from build123d import *

# Parameters (mm, degrees)
SKETCH1_R           = 2.1
BOSS_EXTRUDE1_DEPTH = 1500
FILLET1_R           = 0.5


with BuildPart() as part:
    # Sketch1 → Boss-Extrude1 (new body)
    with BuildSketch(Plane.XY):
        Polygon((-20, -10), (-15.5, -10), (-15.1, -10), (-13.1, -8), (-15.5, -8), (-15.5, -6.560660172), (-12.539339828, -3.6), (-7.460660172, -3.6), (-4.5, -6.560660172), (-4.5, -8), (-6.9, -8), (-4.9, -10), (5.313777138, -10), (7.313777138, -8), (4.5, -8), (4.5, -6.560660172), (7.460660172, -3.6), (12.539339828, -3.6), (15.5, -6.560660172), (15.5, -8), (13.513777138, -8), (15.1, -10), (15.5, -10), (20, -10), (20, -5.5), (20, -5.1), (18, -3.1), (18, -5.5), (16.560660172, -5.5), (13.6, -2.539339828), (13.6, 2.539339828), (16.560660172, 5.5), (18, 5.5), (18, 3.1), (20, 5.1), (20, 5.5), (20, 10), (15.5, 10), (15.1, 10), (13.1, 8), (15.5, 8), (15.5, 6.560660172), (12.539339828, 3.6), (7.460660172, 3.6), (4.5, 6.560660172), (4.5, 8), (7.313777138, 8), (5.313777138, 10), (-4.9, 10), (-6.9, 8), (-4.5, 8), (-4.5, 6.560660172), (-7.460660172, 3.6), (-12.539339828, 3.6), (-15.5, 6.560660172), (-15.5, 8), (-13.1, 8), (-15.1, 10), (-15.5, 10), (-20, 10), (-20, 5.5), (-20, 5.1), (-18, 3.1), (-18, 5.5), (-16.560660172, 5.5), (-13.6, 2.539339828), (-13.6, -2.539339828), (-16.560660172, -5.5), (-18, -5.5), (-18, -3.1), (-20, -5.1), (-20, -5.5), align=None)
        with Locations((-10, 0)):
            Circle(SKETCH1_R, mode=Mode.SUBTRACT)
        with Locations((10, 0)):
            Circle(SKETCH1_R, mode=Mode.SUBTRACT)
        Polygon((3, -5.939339828), (3, -8), (-3, -8), (-3, -5.939339828), (-6.4, -2.539339828), (-6.4, 2.539339828), (-3, 5.939339828), (-3, 8), (3, 8), (3, 5.939339828), (6.4, 2.539339828), (6.4, -2.539339828), align=None, mode=Mode.SUBTRACT)
    extrude(amount=BOSS_EXTRUDE1_DEPTH)

    # Fillet1
    fillet1_edges = [part.edges().sort_by_distance(p)[0] for p in [
        (-20, 10, 750),
        (20, 10, 750),
        (20, -10, 750),
        (-20, -10, 750),
    ]]
    fillet(fillet1_edges, radius=FILLET1_R)


solid = part.part
Check sheet for the modelled part. Datum: model origin and axes. Units: mm. Give positions to 0.01 mm unless a question says otherwise; leave off trailing zeros. Use one line per item in the form item = value.
(1) Section check A-A on z = 994.5. State how many separate pieces and enclosed holes the cut face has, plus the area to 3 significant figures.
Answer block:
separate_pieces = 1
enclosed_holes = 3
area = 283 mm2
(2) Depth check by flat-ended pin: P1, Ø6, axis at y = 5, z = 574, coming from the -X side; P2, Ø4, axis at y = -0.5, z = 590.5, coming from the -X side; P3, Ø5, axis at x = 10.5, z = 1230.5, coming from the -Y side; P4, Ø1.2, axis at y = -4, z = 433.5, coming from the -X side. Enter the tip coordinate at first touch or a pass-through.
Answer block:
P1 = -20
P2 = -13.6
P3 = -4.06
P4 = -19.5
(3) Material ranges on line 1 along Y through (x, z) = (6, 137.5); line 2 along Y through (x, z) = (-10, 946); line 3 along X through (y, z) = (5, 279.5), recorded low to high.
Answer block:
line_1 = -9.31 to -8, -5.06 to -2.94, 2.94 to 5.06, 8 to 9.31
line_2 = -3.6 to -2.1, 2.1 to 3.6
line_3 = -19.9 to -18, -16.06 to -13.94, -6.06 to -3.94, 3.94 to 6.06, 13.94 to 16.06, 18 to 19.9
